Check sheet for the modelled part. Datum: model origin and axes. Units: mm. A direction names the side the tool comes from. Coordinates: 2 decimals unless noted, no trailing zeros. Loops run counter-clockwise (first coordinate to the right, second up) from the corner with the lowest first, then second, coordinate; pieces in that order, holes last. Notation, with made-up numbers: (47, 56) - (73, 56) arc R21 cw to (73, 72) - close; hole circle Ø4 at (-4, 61). An arc over 180 degrees is marked (long way). Write each question's results on one line, items separated by ' | '. Start each with the question number.
1. Thickness scan on line 1 (X direction, y = 2.6, z = 40.75); line 2 (Z direction, x = -21.5, y = 0.3); line 3 (Z direction, x = 16, y = 1.75). Record the ranges inside material, lowest first. Write a range as [from, to].
2. Cross-section at D-D (x = -15). Record the cut outline in (y, z).
3. Cross-section at A-A (y = 2.55). Record the cut outline in (x, z), and give its area (3 significant figures).
4. Cross-section at C-C (x = 22.5). Record the cut outline in (y, z), and give its area (3 significant figures).
5. Gauge pin test, flat end, axial feed: P1, Ø1, axis at x = 1, y = 0.5, coming from the -Z side. Record the tip position at first contact, or that the pin passes through.
6. Tool access check on faces 1 (the face through (-25.434, 1, 45)), 2 (the face through (19.834, 1, 42)). Record the directions out of +Z, -Z, +X, -X, +Y, -Y that give a thin tool (end or side, any length) a straight path to the whole face; none if there is none.
7. Cross-section at B-B (z = 41.5). Record the cut outline in (x, y), and give its area (3 significant figures).
8. Draft check along Z on faces 3 (the face through (-25.103, 1.479, 53.61)), 4 (the face through (0, 1, 51)), 5 (the face through (25.434, 1, 45)), 6 (the face through (-21.36, 1.48, 38.97)). Enter one of: released by +Z, released by -Z, zero draft, split by the parting line, or undercut.
Autodesk Inventor part; units mm, degrees
ref_plane "YZ Plane" through (0, 0, 0) normal (1, 0, 0) x (0, 1, 0)
ref_plane "XZ Plane" through (0, 0, 0) normal (0, 1, 0) x (-1, 0, 0)
ref_plane "XY Plane" through (0, 0, 0) normal (0, 0, 1) x (1, 0, 0)
sketch "Sketch1" plane through (0, 0, 0) normal (0, 1, 0) x (-1, 0, 0)
  circle A0 centre (22.6343, 38) radius 1.6
  circle A1 centre (-22.6343, 38) radius 1.6
  arc A2 (19.8343, 38) -> (25.4343, 38) centre (22.6343, 38) ccw
  arc A3 (-25.4343, 38) -> (-19.8343, 38) centre (-22.6343, 38) ccw
  line L0 (-25.4343, 38) -> (-25.4343, 52.5079)
  line L1 (25.4343, 38) -> (25.4343, 52.5079)
  arc A4 (18.5623, 47.502) -> (-18.5623, 47.502) centre (0, 0) ccw
  line L2 (19.8343, 45.6392) -> (19.8343, 38)
  line L3 (-19.8343, 45.6392) -> (-19.8343, 38)
  arc A5 (24.2494, 54.3343) -> (-24.2494, 54.3343) centre (0, 0) ccw
  arc A6 (25.4343, 52.5079) -> (24.2494, 54.3343) centre (23.4343, 52.5079) ccw
  arc A7 (19.8343, 45.6392) -> (18.5623, 47.502) centre (17.8343, 45.6392) ccw
  arc A8 (-24.2494, 54.3343) -> (-25.4343, 52.5079) centre (-23.4343, 52.5079) ccw
  arc A9 (-18.5623, 47.502) -> (-19.8343, 45.6392) centre (-17.8343, 45.6392) ccw
  point P0 (-25.4343, 53.7898)
  point P1 (25.4343, 53.7898)
  point P2 (19.8343, 46.9851)
  point P3 (-19.8343, 46.9851)
  dimension "d3" = 3.2
  dimension "d4" = 2.8
  dimension "d5" = 2.8
  dimension "d7" = 2
extrude "Extrusion1" add sketch "Sketch1" along normal blind 3
properties part number "Light Sensor Cover"
Established:
1) line 1: [-25.43, -19.83], [19.83, 25.43] | line 2: [35.44, 36.87], [39.13, 55.48] | line 3: [48.43, 57.31]
2) outline: (0, 48.74) - (3, 48.74) - (3, 57.58) - (0, 57.58) - close
3) outline: (-25.43, 38) arc R2.8 ccw to (-19.83, 38) - (-19.83, 45.64) arc R2 cw to (-18.56, 47.5) arc R51 cw to (18.56, 47.5) arc R2 cw to (19.83, 45.64) - (19.83, 38) arc R2.8 ccw to (25.43, 38) - (25.43, 52.51) arc R2 ccw to (24.25, 54.33) arc R59.5 ccw to (-24.25, 54.33) arc R2 ccw to (-25.43, 52.51) - close; hole circle Ø3.2 at (-22.63, 38); hole circle Ø3.2 at (22.63, 38) | area: 544 mm^2
4) outline: (0, 35.2) - (3, 35.2) - (3, 36.41) - (0, 36.41) - close; (0, 39.59) - (3, 39.59) - (3, 55.08) - (0, 55.08) - close | area: 50.1 mm^2
5) P1: z = 50.98
6) face 1: +Z, -Z, -X, +Y, -Y | face 2: -Z, +Y, -Y
7) outline: (-25.43, 0) - (-19.83, 0) - (-19.83, 3) - (-25.43, 3) - close; (19.83, 0) - (25.43, 0) - (25.43, 3) - (19.83, 3) - close | area: 33.6 mm^2
8) face 3: released by +Z | face 4: released by -Z | face 5: zero draft | face 6: undercut
